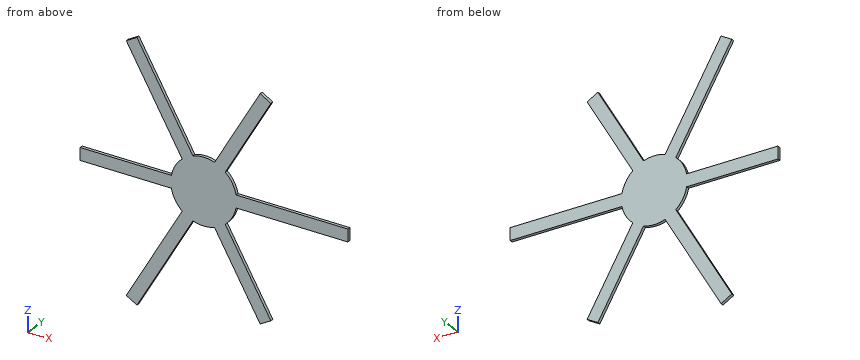
```python
from build123d import *

# Parameters (mm, degrees)
F1_DEPTH = 1.5


with BuildPart() as f1:
    # F0 (on Front) → F1 (new body)
    with BuildSketch(Plane.XZ):
        with BuildLine():
            Line((-60, -3), (-15.716234, -3))
            ThreePointArc((-15.716234, -3), (-13.856406, -8), (-10.456193, -12.110658))
            Line((-10.456193, -12.110658), (-37.598076, -59.121778))
            Line((-37.598076, -59.121778), (-32.401924, -62.121778))
            Line((-32.401924, -62.121778), (-5.260041, -15.110658))
            ThreePointArc((-5.260041, -15.110658), (0, -16), (5.260041, -15.110658))
            Line((5.260041, -15.110658), (27.401924, -53.461524))
            Line((27.401924, -53.461524), (32.598076, -50.461524))
            Line((32.598076, -50.461524), (10.456193, -12.110658))
            ThreePointArc((10.456193, -12.110658), (13.856406, -8), (15.716234, -3))
            Line((15.716234, -3), (70, -3))
            Line((70, -3), (70, 3))
            Line((70, 3), (15.716234, 3))
            ThreePointArc((15.716234, 3), (13.856406, 8), (10.456193, 12.110658))
            Line((10.456193, 12.110658), (32.598076, 50.461524))
            Line((32.598076, 50.461524), (27.401924, 53.461524))
            Line((27.401924, 53.461524), (5.260041, 15.110658))
            ThreePointArc((5.260041, 15.110658), (0, 16), (-5.260041, 15.110658))
            Line((-5.260041, 15.110658), (-32.401924, 62.121778))
            Line((-32.401924, 62.121778), (-37.598076, 59.121778))
            Line((-37.598076, 59.121778), (-10.456193, 12.110658))
            ThreePointArc((-10.456193, 12.110658), (-13.856406, 8), (-15.716234, 3))
            Line((-15.716234, 3), (-60, 3))
            Line((-60, 3), (-60, -3))
        make_face()
    extrude(amount=F1_DEPTH)


solid = f1.part
```
CAD build for the part. Positions are in the model's coordinates, mm. Coordinates: 2 decimals unless noted, no trailing zeros. Write each loop counter-clockwise with the first axis right and the second up, starting at its lowest first coordinate (ties: lowest second). Pieces come first, ordered by that corner, then holes.
(1) Cut at D-D, the plane x = -47. List the corners of the cut face in (y, z).
(2) Cut at C-C, the plane z = 17.5. List the corners of the cut face in (x, y), and give its area (3 significant figures).
(3) Cut at A-A, the plane y = -0.65. List the corners of the cut face in (x, z).
(4) Flat gauge pins, fed straight in: pin 1 (0.8 mm diameter, centred on x = -44, y = -1, fed in from -Z); pin 2 (2 mm diameter, centred on x = 34, z = -48.5, fed in from -Y). Where does each tip first touch, or does it go through?
(5) Cut at B-B, the plane x = -30. List the corners of the cut face in (y, z).
(6) Drill centre lines: probe 1 along Z at (x, y) = (30, -0.3); probe 2 along Z at (x, y) = (-21, -0.1); probe 3 along Z at (x, y) = (-45, -1.4). Where is each one in solid material? Low to high.
Geometry says:
1. outline: (-1.5, -3) - (0, -3) - (0, 3) - (-1.5, 3) - close
2. outline: (-13.57, -1.5) - (-6.64, -1.5) - (-6.64, 0) - (-13.57, 0) - close; (6.64, -1.5) - (13.57, -1.5) - (13.57, 0) - (6.64, 0) - close
2. area: 20.8 mm2
3. outline: (-60, -3) - (-15.72, -3) arc R16 ccw to (-10.46, -12.11) - (-37.6, -59.12) - (-32.4, -62.12) - (-5.26, -15.11) arc R16 ccw to (5.26, -15.11) - (27.4, -53.46) - (32.6, -50.46) - (10.46, -12.11) arc R16 ccw to (15.72, -3) - (70, -3) - (70, 3) - (15.72, 3) arc R16 ccw to (10.46, 12.11) - (32.6, 50.46) - (27.4, 53.46) - (5.26, 15.11) arc R16 ccw to (-5.26, 15.11) - (-32.4, 62.12) - (-37.6, 59.12) - (-10.46, 12.11) arc R16 ccw to (-15.72, 3) - (-60, 3) - close
4. pin 1: stops at z = -3
4. pin 2: passes through
5. outline: (-1.5, -57.96) - (0, -57.96) - (0, -45.96) - (-1.5, -45.96) - close; (-1.5, -3) - (0, -3) - (0, 3) - (-1.5, 3) - close; (-1.5, 45.96) - (0, 45.96) - (0, 57.96) - (-1.5, 57.96) - close
6. probe 1: z = -51.96 to -45.96, -3 to 3, 45.96 to 51.96
6. probe 2: z = -42.37 to -30.37, -3 to 3, 30.37 to 42.37
6. probe 3: z = -3 to 3
